Read the model definition and answer for the solid it produces. Units are mm, in the model's axes. A direction names the side the tool comes from. Give positions to 0.01 mm unless a question says otherwise; leave off trailing zeros. Order: outer loops, then holes, each group sorted by start corner. A loop starts at its lowest first (then second) coordinate and runs counter-clockwise, first axis right, second up.
```python
from build123d import *

# Parameters (mm, degrees)
F1_DEPTH = 25
F2_W     = 150.479242
F2_H     = 25
F3_DEPTH = 200
F5_DEPTH = 25.001
F7_DEPTH = 26


with BuildPart() as f1:
    # F0 (on Top) → F1 (new body)
    with BuildSketch(Plane.XY):
        with BuildLine():
            Line((-75.239621, 126.136482), (-75.239621, 0))
            ThreePointArc((-75.239621, 0), (0, -46.155653), (75.239621, 0))
            Line((75.239621, 0), (75.239621, 126.136482))
            Line((75.239621, 126.136482), (-75.239621, 126.136482))
        make_face()
    extrude(amount=-F1_DEPTH)

    # F2 (on face) → F3 (join)
    with BuildSketch(Plane.XY):
        with Locations((0, 113.636482)):
            Rectangle(F2_W, F2_H)
    extrude(amount=F3_DEPTH)

    # F4 (on face) → F5 (cut, through all)
    with BuildSketch(Plane.XZ.offset(-101.136482)):
        with BuildLine():
            Line((-24.937427, 200), (-24.937427, 129.60729))
            ThreePointArc((-24.937427, 129.60729), (0, 104.669863), (24.937427, 129.60729))
            Line((24.937427, 129.60729), (24.937427, 200))
            Line((24.937427, 200), (-24.937427, 200))
        make_face()
    extrude(amount=-F5_DEPTH, mode=Mode.SUBTRACT)

    # F6 (on face) → F7 (cut)
    with BuildSketch(Plane.YZ.offset(75.239621)):
        Polygon((76.136482, -25), (126.136482, -25), (126.136482, 25), (101.136482, 25), (101.136482, 0), (76.136482, 0), align=None)
    extrude(amount=-F7_DEPTH, mode=Mode.SUBTRACT)


solid = f1.part
```
1) The part is cut by section B-B on z = 18. Determine the outline of the cut face in (x, y).
Final values:
outline: (-75.24, 101.14) - (49.24, 101.14) - (49.24, 126.14) - (-75.24, 126.14) - close
2) The part is cut by section C-C on x = 0. Determine the outline of the cut face in (y, z), and give its area (3 significant figures).
Final values:
outline: (-46.16, -25) - (126.14, -25) - (126.14, 104.67) - (101.14, 104.67) - (101.14, 0) - (-46.16, 0) - close
area: 6,920 mm2
3) For a pull along X with two mould halves and no side action, classify faces 1 (the face through (-0.548, 113.461, 104.676)), 2 (the face through (62, 114, 25)), 3 (the face through (75.24, 113, 111)) as released by +X, released by -X, zero draft, split by the parting line, or undercut.
Final values:
face 1: undercut
face 2: zero draft
face 3: released by +X
4) A tool of negligible diameter and unlimited length cuts with its end or side. For faces 4 (the face through (62, 76.136, -12)), 5 (the face through (49.24, 106, -5)), 6 (the face through (-1, 101.136, 99)), 7 (the face through (24.937, 113, 164)), from which of +Z, -Z, +X, -X, +Y, -Y can it reach the whole face along a straight path? Write none if from no direction.
Final values:
face 4: +Z, -Z, +X, +Y
face 5: -Z, +X, +Y
face 6: +Z, +X, -X, -Y
face 7: +Z, +Y, -Y
5) The part is cut by section D-D on y = 53. Determine the outline of the cut face in (x, z).
Final values:
outline: (-75.24, -25) - (75.24, -25) - (75.24, 0) - (-75.24, 0) - close
6) Given pin 1 (12.5 mm diameter, centred on x = 66, z = -15.5, fed in from +Y); pin 2 (6 mm diameter, centred on x = 30.5, z = 175, fed in from -Y); pin 3 (7.5 mm diameter, centred on x = 68.5, y = 119, fed in from -Z), each flat-ended and moving along its own axis, determine where each tip first touches the part or whether it passes through.
Final values:
pin 1: stops at y = 76.14
pin 2: stops at y = 101.14
pin 3: stops at z = 25
7) The part is cut by section A-A on z = 136. Determine the outline of the cut face in (x, y).
Final values:
outline: (-75.24, 101.14) - (-24.94, 101.14) - (-24.94, 126.14) - (-75.24, 126.14) - close; (24.94, 101.14) - (75.24, 101.14) - (75.24, 126.14) - (24.94, 126.14) - close
8) Consider L1, parallel to X at y = 108, z = 175.5; L2, parallel to Y at x = -39, z = 164; L3, parallel to Z at x = -15, y = 33.5. Determine where each line is inside the solid, lowest interval first.
Final values:
L1: x = -75.24 to -24.94, 24.94 to 75.24
L2: y = 101.14 to 126.14
L3: z = -25 to 0
